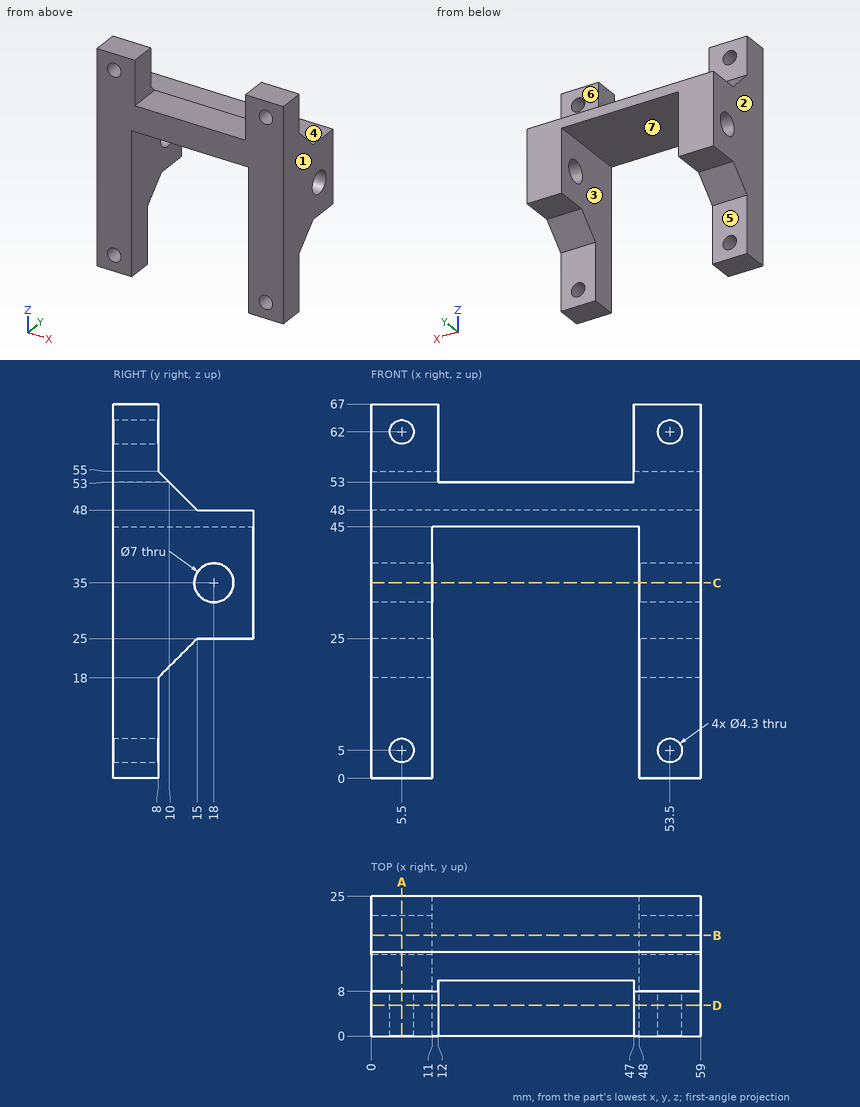
Design review of the part shown in the three views and the two pictorial views. Dimensions are in mm from the part's minimum x, y and z. A direction names the side the tool comes from. Round coordinates to 2 decimals unless told otherwise and drop trailing zeros. Loops run counter-clockwise (first coordinate to the right, second up) from the corner with the lowest first, then second, coordinate; pieces in that order, holes last.
Q1. Mouldability with a two-part tool opening along X and no side actions: class the marked faces 1, 2, 3 and 4 as +X half, -X half, draft (parallel to the pull), parting line (faces both ways), or undercut.
Result sheet:
face 1: +X half
face 2: -X half
face 3: undercut
face 4: draft
Q2. Add section C-C on z = 35. Write out the cut boundary in (x, y), plus the area to 3 significant figures.
Result sheet:
outline: (0, 0) - (11, 0) - (11, 14.5) - (0, 14.5) - close; (0, 21.5) - (11, 21.5) - (11, 25) - (0, 25) - close; (48, 0) - (59, 0) - (59, 14.5) - (48, 14.5) - close; (48, 21.5) - (59, 21.5) - (59, 25) - (48, 25) - close
area: 396 mm2
Q3. To check wall thickness, follow line 1 along Z through (x, y) = (5.5, 4.5); line 2 along X through (y, z) = (6.25, 18.5); line 3 along X through (y, z) = (5.5, 62). State the ranges of each line that lie inside material, in increasing order.
Result sheet:
line 1: z = 0 to 2.85, 7.15 to 59.85, 64.15 to 67
line 2: x = 0 to 11, 48 to 59
line 3: x = 0 to 3.35, 7.65 to 12, 47 to 51.35, 55.65 to 59
Q4. Add section B-B on y = 18. Write out the cut boundary in (x, z), plus the area to 3 significant figures.
Result sheet:
outline: (0, 25) - (11, 25) - (11, 31.5) - (0, 31.5) - close; (0, 38.5) - (11, 38.5) - (11, 45) - (48, 45) - (48, 38.5) - (59, 38.5) - (59, 48) - (0, 48) - close; (48, 25) - (59, 25) - (59, 31.5) - (48, 31.5) - close
area: 463 mm2
Q5. Add section A-A on x = 5.5. Write out the cut boundary in (y, z), plus the area to 3 significant figures.
Result sheet:
outline: (0, 0) - (8, 0) - (8, 2.85) - (0, 2.85) - close; (0, 7.15) - (8, 7.15) - (8, 18) - (15, 25) - (25, 25) - (25, 48) - (15, 48) - (8, 55) - (8, 59.85) - (0, 59.85) - close; (0, 64.15) - (8, 64.15) - (8, 67) - (0, 67) - close; hole circle Ø7 at (18, 35)
area: 869 mm2
Q6. Add section D-D on y = 5.5. Write out the cut boundary in (x, z), plus the area to 3 significant figures.
Result sheet:
outline: (0, 0) - (11, 0) - (11, 45) - (48, 45) - (48, 0) - (59, 0) - (59, 67) - (47, 67) - (47, 53) - (12, 53) - (12, 67) - (0, 67) - close; hole circle Ø4.3 at (5.5, 5); hole circle Ø4.3 at (5.5, 62); hole circle Ø4.3 at (53.5, 5); hole circle Ø4.3 at (53.5, 62)
area: 1,740 mm2
Q7. Machinability: for the marked faces 5, 6 and 7, which of the approach directions +Z, -Z, +X, -X, +Y, -Y give a long, thin tool a straight path to every point of the face, cutting with its end or side? Answer none if there is none.
Result sheet:
face 5: -Z, +X, -X, +Y
face 6: +Z, +X, -X, +Y
face 7: -Z, +Y, -Y
Q8. Insertion check: pin 1 Ø3.5 at (x, z) = (3.5, 63) entering from +Y; pin 2 Ø6 at (x, y) = (6, 17.5) entering from -Z; pin 3 Ø4 at (x, y) = (52.5, 15.5) entering from +Z. Each pin has a flat end and moves straight along its axis. Give the tip position at first contact, or say it passes through.
Result sheet:
pin 1: stops at y = 8
pin 2: stops at z = 24.5
pin 3: stops at z = 49.5
